For this review, take the finished solid that the model builds, in its own axes (mm). Face numbers are marked on the shaded views. A direction names the side the tool comes from. Give positions to 0.01 mm unless a question says otherwise; leave off trailing zeros. Write each loop counter-clockwise with the first axis right and the second up, starting at its lowest first coordinate (ties: lowest second). Pieces come first, ordered by that corner, then holes.
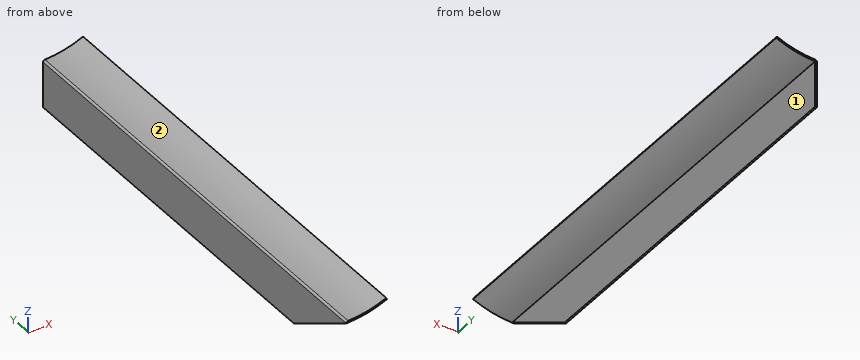
from build123d import *

# Parameters (mm, degrees)
BASE_FLANGE1_DEPTH = 381
CUT_EXTRUDE3_DEPTH = 384.680964443


# Read off the part's stored shape, not the designer's step: Base-Flange1
with BuildPart() as part:
    # Base-Flange1 outline → Base-Flange1 (new body)
    with BuildSketch(Plane(origin=(0, 0, 0), x_dir=(1, 0, 0), z_dir=(0, 1, 0))):
        with BuildLine():
            Line((-19.546720325, -22.80599753), (-19.546720325, 15.29400247))
            Line((-19.546720325, 15.29400247), (-21.070720325, 15.29400247))
            Line((-21.070720325, 15.29400247), (-21.070720325, -22.80599753))
            ThreePointArc((-21.070720325, -22.80599753), (-20.617741894, -23.916410543), (-19.517313006, -24.393131405))
            ThreePointArc((-19.517313006, -24.393131405), (-19.511747403, -24.393260722), (-19.506182287, -24.393409555))
            ThreePointArc((-19.506182287, -24.393409555), (-3.280067744, -26.452317081), (12.23727224, -31.623202224))
            Line((12.23727224, -31.623202224), (12.857840422, -30.231271503))
            ThreePointArc((12.857840422, -30.231271503), (-2.941633017, -24.966370266), (-19.462767824, -22.870028058))
            ThreePointArc((-19.462767824, -22.870028058), (-19.47367545, -22.869736345), (-19.484584032, -22.869482885))
            ThreePointArc((-19.484584032, -22.869482885), (-19.528601188, -22.85041405), (-19.546720325, -22.80599753))
        make_face()
    extrude(amount=BASE_FLANGE1_DEPTH)

    # Sketch5 → Cut-Extrude3 (cut, through all)
    with BuildSketch(Plane(origin=(-19.546720325, 0, 0), x_dir=(0, 0, -1), z_dir=(1, 0, 0))):
        Polygon((-22.80599753, 0), (15.29400247, 65.991135768), (15.29400247, 0), align=None)
    extrude(amount=-CUT_EXTRUDE3_DEPTH, mode=Mode.SUBTRACT)


solid = part.part
(1) We need section C-C (x = -12). Write out the cut boundary in (y, z), and give its area (3 significant figures).
(2) Clearance check with flat-ended pins moving along their axes: pin 1 Ø12 at (x, y) = (-6, 168) entering from +Z; pin 2 Ø4 at (x, y) = (3, 117) entering from -Z; pin 3 Ø6 at (x, y) = (0, 338.5) entering from +Z; pin 4 Ø10 at (y, z) = (50, 23.5) entering from -X. State where each tip first meets the part, or that it passes through.
(3) Tool access review of the marked faces 1 and 2: name each direction out of +Z, -Z, +X, -X, +Y, -Y from which nothing blocks a thin tool from reaching the whole face with its end or side.
(4) We need section B-B (z = 18). Write out the cut boundary in (x, y).
(5) For L1, parallel to X at y = 318.5, z = 3.5; L2, parallel to Z at x = 8, y = 27; L3, parallel to Z at x = -11, y = 263, list the stretches that pass through material, from the lowest coordinate up.
The answers:
1. outline: (0, 23.41) - (381, 23.41) - (381, 24.95) - (0, 24.95) - close
1. area: 585 mm2
2. pin 1: stops at z = 27.27
2. pin 2: stops at z = 25.96
2. pin 3: stops at z = 28.14
2. pin 4: stops at x = -21.07
3. face 1: -Z, +X, +Y, -Y
3. face 2: +Z, -X, +Y, -Y
4. outline: (-21.07, 8.32) - (-19.55, 8.32) - (-19.55, 381) - (-21.07, 381) - close
5. L1: x = -21.07 to -19.55
5. L2: z = 28.24 to 29.87
5. L3: z = 23.53 to 25.07
